Work out the finished part from the listing and answer in its coordinate system (mm). A direction names the side the tool comes from. Round coordinates to 2 decimals unless told otherwise and drop trailing zeros. Order: outer loops, then holes, each group sorted by start corner. A loop starts at its lowest first (then second) coordinate and runs counter-clockwise, first axis right, second up. Notation, with made-up numbers: M 74,63 L 91,63 A14 ccw 91,88 Z; hole C 53.25,86.25 d2. An arc over 180 degrees is marked long. Return JSON: item names as keys, results as strings.
from build123d import *

# Parameters (mm, degrees)
SKETCH1_W           = 128.5875
SKETCH1_H           = 144.4625
BOSS_EXTRUDE1_DEPTH = 61.07176
SHELL1_T            = 6.35
SKETCH2_R           = 8.73125
SKETCH2_R_2         = 19.84375
SKETCH2_W           = 45.72
SKETCH2_H           = 63.1825
SKETCH2_W_2         = 69.215
SKETCH2_H_2         = 23.8125
CUT_EXTRUDE1_DEPTH  = 126.344509202
SKETCH3_W           = 31.75
SKETCH3_H           = 66.675
CUT_EXTRUDE2_DEPTH  = 173.82051492


with BuildPart() as part:
    # Sketch1 → Boss-Extrude1 (new body)
    with BuildSketch(Plane.XY):
        Rectangle(SKETCH1_W, SKETCH1_H)
    extrude(amount=-BOSS_EXTRUDE1_DEPTH)

    # Shell1
    shell1_openings = [part.faces().sort_by_distance(p)[0] for p in [
        (0, 0, -61.07176),
    ]]
    offset(amount=SHELL1_T, openings=shell1_openings, kind=Kind.INTERSECTION)

    # Sketch2 → Cut-Extrude1 (cut, through all)
    with BuildSketch(Plane.XY.offset(6.35)):
        with Locations((-31.75, 50.8)):
            Circle(SKETCH2_R)
        with Locations((-31.75, 9.525)):
            Circle(SKETCH2_R_2)
        with Locations((26.19375, 25.4)):
            Rectangle(SKETCH2_W, SKETCH2_H)
        with Locations((11.90625, -41.275)):
            Rectangle(SKETCH2_W_2, SKETCH2_H_2)
    extrude(amount=-CUT_EXTRUDE1_DEPTH, mode=Mode.SUBTRACT)

    # Sketch3 → Cut-Extrude2 (cut, through all)
    with BuildSketch(Plane(origin=(70.64375, 0, 0), x_dir=(0, 0, -1), z_dir=(1, 0, 0))):
        with Locations((31.39694, -13.43025)):
            Rectangle(SKETCH3_W, SKETCH3_H)
    extrude(amount=-CUT_EXTRUDE2_DEPTH, mode=Mode.SUBTRACT)


solid = part.part
Item 1: This flat-tipped pin is pushed along its axis until it touches: pin 1 (1.5 mm diameter, centred on x = -31.5, y = 42.5, fed in from -Z). Where does it stop, or does it pass through?
Output:
{"pin 1": "stops at z = 0"}
Item 2: Which of the six approach directions +Z, -Z, +X, -X, +Y, -Y give full straight-line access (tool end or side, diameter ignored) to faces 1 (the flat face through (3.334, 25, 3)), 2 (the flat face through (-64.294, -1, -50)), 3 (the flat face through (68, -14, -47.272))?
Output:
{"face 1": "+Z, -Z", "face 2": "-Z", "face 3": "+X, -X"}
Item 3: Find section A-A (y = -22). Determine the outline of the cut face in (x, z), plus the area to 3 significant figures.
Output:
{"outline": "M -70.64,-61.07 L -64.29,-61.07 L -64.29,-47.27 L -70.64,-47.27 Z; M -70.64,-15.52 L -64.29,-15.52 L -64.29,0 L 64.29,0 L 64.29,-15.52 L 70.64,-15.52 L 70.64,6.35 L -70.64,6.35 Z; M 64.29,-61.07 L 70.64,-61.07 L 70.64,-47.27 L 64.29,-47.27 Z", "area": "1,270 mm^2"}
Item 4: Find section B-B (x = 15). Determine the outline of the cut face in (y, z), plus the area to 3 significant figures.
Output:
{"outline": "M -78.58,-61.07 L -72.23,-61.07 L -72.23,0 L -53.18,0 L -53.18,6.35 L -78.58,6.35 Z; M -29.37,0 L -6.19,0 L -6.19,6.35 L -29.37,6.35 Z; M 56.99,0 L 72.23,0 L 72.23,-61.07 L 78.58,-61.07 L 78.58,6.35 L 56.99,6.35 Z", "area": "1,220 mm^2"}
Item 5: Find section C-C (z = -26). Determine the outline of the cut face in (x, y).
Output:
{"outline": "M -70.64,-78.58 L 70.64,-78.58 L 70.64,-46.77 L 64.29,-46.77 L 64.29,-72.23 L -64.29,-72.23 L -64.29,-46.77 L -70.64,-46.77 Z; M -70.64,19.91 L -64.29,19.91 L -64.29,72.23 L 64.29,72.23 L 64.29,19.91 L 70.64,19.91 L 70.64,78.58 L -70.64,78.58 Z"}
Item 6: Consider line 1 along Y through (x, z) = (-31.75, 5); line 2 along X through (y, z) = (49.5, -11.5); line 3 along Y through (x, z) = (-28.5, -18). Determine where each line is inside the solid, lowest interval first. Write a range as [from, to].
Output:
{"line 1": "y = [-78.58, -10.32], [29.37, 42.07], [59.53, 78.58]", "line 2": "x = [-70.64, -64.29], [64.29, 70.64]", "line 3": "y = [-78.58, -72.23], [72.23, 78.58]"}
Item 7: Find section D-D (z = -53.5). Determine the outline of the cut face in (x, y).
Output:
{"outline": "M -70.64,-78.58 L 70.64,-78.58 L 70.64,78.58 L -70.64,78.58 Z; hole M -64.29,-72.23 L 64.29,-72.23 L 64.29,72.23 L -64.29,72.23 Z"}
Item 8: The mould has two halves that part along X. Classify faces 4 (the flat face through (46.514, -41, 3)), 5 (the flat face through (70.644, -1, -12)), 6 (the flat face through (-1, 78.581, -27)): pulls with the +X half, pulls with the -X half, needs draft (parallel to the pull), parting line crosses it, or undercut.
Output:
{"face 4": "undercut", "face 5": "pulls with the +X half", "face 6": "needs draft"}
